Here's how the part is built. I have some questions about the finished solid (model axes, mm). Face numbers are marked on the shaded views. Round coordinates to 2 decimals unless told otherwise and drop trailing zeros. Write each loop counter-clockwise with the first axis right and the second up, starting at its lowest first coordinate (ties: lowest second). Pieces come first, ordered by that corner, then holes. Notation, with made-up numbers: (34.25, -18.75) - (69.25, -18.75) arc R30 ccw to (69.25, 18.25) - close; hole circle Ø8 at (34, 30). An arc over 180 degrees is marked (long way). Use one line per item in the form item = value. Start each with the question number.
1. I want a section at A-A, the plane y = 0. List the corners of the cut face in (x, z) for me.
2. I want a section at C-C, the plane x = -0.75. List the corners of the cut face in (y, z) for me.
3. I want a section at D-D, the plane z = 6.25. List the corners of the cut face in (x, y) for me, plus the area to 3 significant figures.
4. If I drill on line 1 along Z through (x, y) = (0, 9); line 2 along Y through (x, z) = (0, 3.5); line 3 along Y through (x, z) = (-0.25, 8.75), over which ranges is the centre line in solid material (lowest first)?
5. I want a section at B-B, the plane z = 2.5. List the corners of the cut face in (x, y) for me, plus the area to 3 significant figures.
6. We'd pull the mould along Z, two halves only. Please class the marked faces 1, 2, 3 and 4: +Z half, -Z half, draft (parallel to the pull), parting line (faces both ways), or undercut.
7. Will these pins go through, and if not, where does the flat tip stop? pin 1 (4 mm diameter, centred on x = 0.5, z = 4, fed in from -Y); pin 2 (6 mm diameter, centred on x = 5.5, z = 4, fed in from -Y); pin 3 (1 mm diameter, centred on y = -3, z = 7, fed in from +X); pin 4 (1 mm diameter, centred on x = -0.5, y = -1.5, fed in from +Z).
```python
from build123d import *

# Parameters (mm, degrees)
SKETCH_1_R          = 10
EXTRUDE_1_DEPTH     = 10
SKETCH_2_R          = 2.2
CUT_EXTRUDE_2_DEPTH = 10
CUT_EXTRUDE_3_DEPTH = 10
SKETCH_5_R          = 1.65
CUT_EXTRUDE_4_DEPTH = 10
CUT_EXTRUDE_START   = -3.6
CUT_EXTRUDE_5_DEPTH = 2.8


with BuildPart() as part:
    # Эскиз1 → Бобышка-Вытянуть1 (new body)
    with BuildSketch(Plane.XY):
        Circle(SKETCH_1_R)
    extrude(amount=EXTRUDE_1_DEPTH)

    # Эскиз2 → Вырез-Вытянуть2 (cut)
    with BuildSketch(Plane(origin=(0, 0, 0), x_dir=(-1, 0, 0), z_dir=(0, 0, -1))):
        Circle(SKETCH_2_R)
    extrude(amount=-CUT_EXTRUDE_2_DEPTH, mode=Mode.SUBTRACT)

    # Sketch 4 → Вырез-Вытянуть3 (cut)
    with BuildSketch(Plane(origin=(10, 6.4, 7.9), x_dir=(0, -0.4287444523171483, -0.9034258102397056), z_dir=(1, 0, 0))):
        Polygon((0, 0), (5.33021228, 2.529592269), (6.530696747, 0), (1.200484466, -2.529592269), align=None)
    extrude(amount=-CUT_EXTRUDE_3_DEPTH, mode=Mode.SUBTRACT)

    # Эскиз5 → Вырез-Вытянуть4 (cut)
    with BuildSketch(Plane(origin=(0, 10, 0), x_dir=(1, 0, 0), z_dir=(0, 1, 0))):
        with Locations(Location((0, -5, 0), (0, 0, 270))):
            Circle(SKETCH_5_R)
    extrude(amount=-CUT_EXTRUDE_4_DEPTH, mode=Mode.SUBTRACT)

    # Эскиз6 → Вырез-Вытянуть5 (cut)
    with BuildSketch(Plane(origin=(0, 10, 0), x_dir=(1, 0, 0), z_dir=(0, 1, 0)).offset(CUT_EXTRUDE_START)):
        Polygon((-1.703183294, -2.05), (-3.406366588, -5), (-1.703183294, -7.95), (1.703183294, -7.95), (3.406366588, -5), (1.703183294, -2.05), align=None)
    extrude(amount=-CUT_EXTRUDE_5_DEPTH, mode=Mode.SUBTRACT)


solid = part.part
```
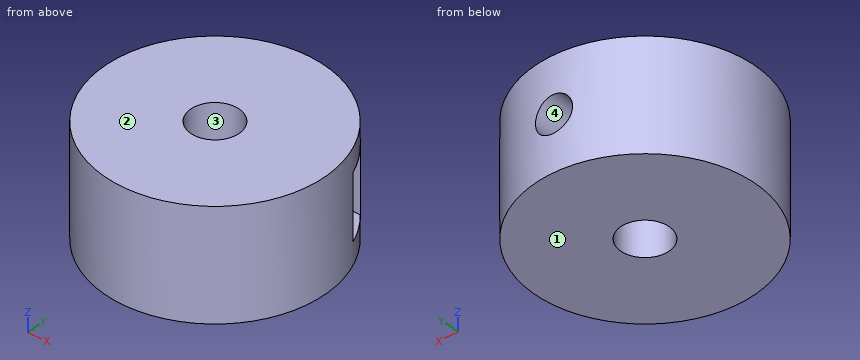
Model answer:
q1.outline = (-10, 0) - (-2.2, 0) - (-2.2, 10) - (-10, 10) - close; (2.2, 0) - (10, 0) - (10, 10) - (2.2, 10) - close
q2.outline = (-9.97, 0) - (-2.07, 0) - (-2.07, 10) - (-9.97, 10) - close; (2.07, 0) - (9.97, 0) - (9.97, 3.53) - (6.4, 3.53) - (6.4, 2.05) - (3.6, 2.05) - (3.6, 3.53) - (2.07, 3.53) - close; (2.07, 6.47) - (3.6, 6.47) - (3.6, 7.95) - (6.4, 7.95) - (6.4, 6.47) - (9.97, 6.47) - (9.97, 10) - (2.07, 10) - close
q3.outline = (-2.68, 3.6) - (-2.68, 6.4) - (-1.08, 6.4) - (-1.08, 9.94) arc R10 ccw (long way) to (9.33, 3.6) - (1.08, 3.6) - (1.08, 1.92) arc R2.2 cw (long way) to (-1.08, 1.92) - (-1.08, 3.6) - close; (1.08, 6.4) - (7.68, 6.4) arc R10 ccw to (1.08, 9.94) - close
q3.area = 256 mm2
q4.line_1 = 0 to 3.35, 6.65 to 10
q4.line_2 = -10 to -2.2
q4.line_3 = -10 to -2.19, 2.19 to 10
q5.outline = (-1.96, 3.6) - (-1.96, 6.4) - (7.68, 6.4) arc R10 ccw (long way) to (9.33, 3.6) - close; hole circle Ø4.4 at (0, 0)
q5.area = 269 mm2
q6.face_1 = -Z half
q6.face_2 = +Z half
q6.face_3 = draft
q6.face_4 = undercut
q7.pin_1 = -10
q7.pin_2 = -9.68
q7.pin_3 = 9.68
q7.pin_4 = through
